CAD build for the part. Positions are in the model's coordinates, mm. A direction names the side the tool comes from. Coordinates: 2 decimals unless noted, no trailing zeros. Write each loop counter-clockwise with the first axis right and the second up, starting at its lowest first coordinate (ties: lowest second). Pieces come first, ordered by that corner, then holes. Notation, with made-up numbers: (-1.5, 81) - (20.5, 81) arc R25 cw to (20.5, 93) - close; hole circle Ø1 at (-28, 18). An arc over 180 degrees is marked (long way). One line per question, with ' | ' between items. Start each with the question number.
1. Which spindle directions (+Z, -Z, +X, -X, +Y, -Y) get a long thin tool onto all of the face, cutting with end or side? Do faces 1 (the flat face through (0, 0, 184.15)), 2 (the cylindrical face through (-3.345, 25.475, 155.175)). Say none if no direction does.
2. Probe line 1 (Z direction, x = -26.5, y = -7.5); line 2 (X direction, y = 15.5, z = 165.5); line 3 (X direction, y = -9, z = 164.5). List the from-to ranges inside material, lowest first.
3. Band-saw the part on A-A, the plane y = 0. Write the cut outline in (x, z), then the cut area to 3 significant figures.
4. Band-saw the part on C-C, the plane z = 151. Write the cut outline in (x, y).
5. Flat gauge pin, fed straight in: P1, Ø12, axis at x = -10.5, z = 142.5, coming from the +Y side. Where does the tip first touch, or does it go through?
6. Band-saw the part on B-B, the plane x = -6.5. Write the cut outline in (y, z).
from build123d import *

# Parameters (mm, degrees)
F0_R     = 29.8738984084
F1_DEPTH = 101.6
F3_W     = 84.1787829995
F3_H     = 53.359227255
F4_DEPTH = 127
F5_R     = 25.6938626455
F6_DEPTH = 57.15


with BuildPart() as f1:
    # F0 (on Top) → F1 (new body)
    with BuildSketch(Plane.XY):
        Circle(F0_R)
    extrude(amount=F1_DEPTH)


with BuildPart() as f4:
    # F3 (on Top) → F4 (new body)
    with BuildSketch(Plane.XY):
        with Locations((-0.8001253009, 0.2058306709)):
            Rectangle(F3_W, F3_H)
    extrude(amount=F4_DEPTH)

    # F5 (on face) → F6 (join)
    with BuildSketch(Plane.XY.offset(127)):
        Circle(F5_R)
    extrude(amount=F6_DEPTH)


solid = f4.part
Filled in:
1) face 1: +Z, +X, -X, +Y, -Y | face 2: +Z
2) line 1: z = 0 to 127 | line 2: x = -20.49 to 20.49 | line 3: x = -24.07 to 24.07
3) outline: (-42.89, 0) - (41.29, 0) - (41.29, 127) - (25.69, 127) - (25.69, 184.15) - (-25.69, 184.15) - (-25.69, 127) - (-42.89, 127) - close | area: 13,600 mm²
4) outline: circle Ø51.39 at (0, 0)
5) P1: stops at y = 25.3
6) outline: (-26.47, 0) - (26.89, 0) - (26.89, 127) - (24.86, 127) - (24.86, 184.15) - (-24.86, 184.15) - (-24.86, 127) - (-26.47, 127) - close
